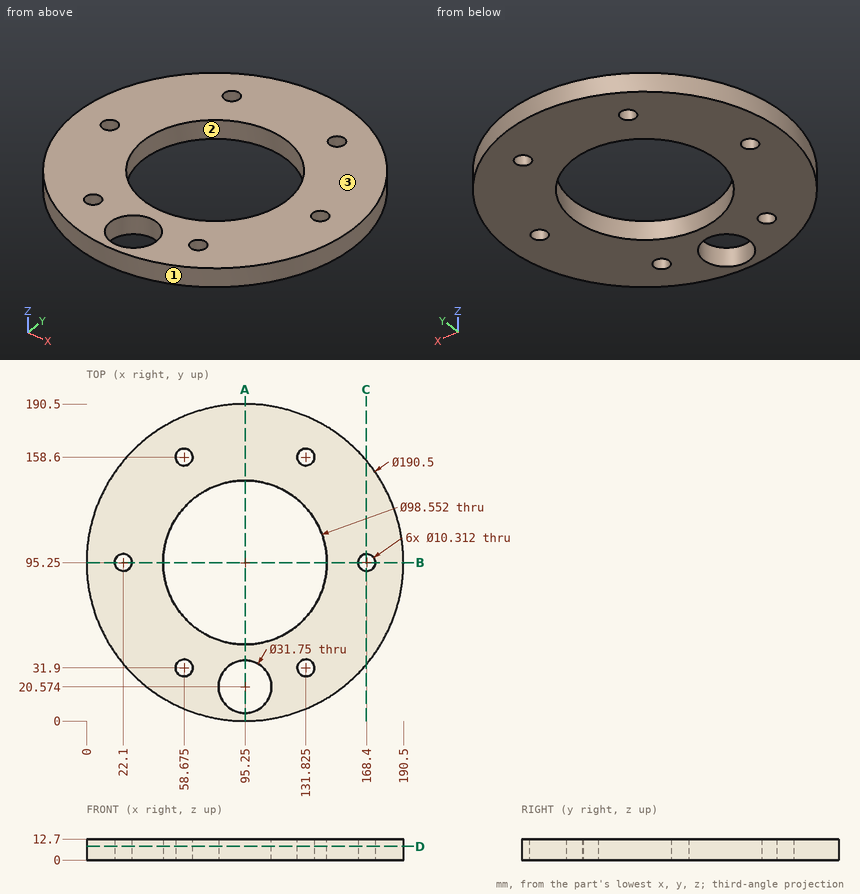
Could you check a few things on this drawing? It's one solid part, dimensions in mm from its lowest x, y, z. Give positions to 0.01 mm unless a question says otherwise; leave off trailing zeros. Loops run counter-clockwise (first coordinate to the right, second up) from the corner with the lowest first, then second, coordinate; pieces in that order, holes last. Notation, with made-up numbers: M -36.75,-37.75 L -28.75,-37.75 A19 cw -28.75,-33.75 Z; hole C 48.25,-33.5 d5. An arc over 180 degrees is marked long. Return JSON: item names as keys, results as strings.
Item 1: Thinking about a two-plate mould opening in X: for the marked faces 1, 2 and 3, which applies, released by +X, released by -X, zero draft, split by the parting line, or undercut?
A:
{"face 1": "split by the parting line", "face 2": "undercut", "face 3": "zero draft"}
Item 2: Imagine slicing it at A-A on x = 95.25. List the corners of the cut face in (y, z) for me.
A:
{"outline": "M 0,0 L 4.7,0 L 4.7,12.7 L 0,12.7 Z; M 36.45,0 L 45.97,0 L 45.97,12.7 L 36.45,12.7 Z; M 144.53,0 L 190.5,0 L 190.5,12.7 L 144.53,12.7 Z"}
Item 3: Imagine slicing it at C-C on x = 168. List the corners of the cut face in (y, z) for me.
A:
{"outline": "M 33.77,0 L 90.11,0 L 90.11,12.7 L 33.77,12.7 Z; M 100.39,0 L 156.73,0 L 156.73,12.7 L 100.39,12.7 Z"}
Item 4: I'm going to push flat-ended pins straight in: pin 1 Ø6 at (x, z) = (124, 2) entering from -Y; pin 2 Ø5 at (y, z) = (112, 11) entering from -X; pin 3 Ø3 at (x, z) = (57, 9) entering from -Y (1 decimal). Where does each tip first touch, or does it pass through?
A:
{"pin 1": "stops at y = 3.55", "pin 2": "stops at x = 1.07", "pin 3": "stops at y = 7.4"}
Item 5: Imagine slicing it at D-D on z = 8.25. State how many separate pieces and enclosed holes the cut face has, then the cut area to 3 significant figures.
A:
{"separate pieces": "1", "enclosed holes": "8", "area": "19,600 mm^2"}
Item 6: Imagine slicing it at B-B on y = 95.25. List the corners of the cut face in (x, z) for me, then the cut area to 3 significant figures.
A:
{"outline": "M 0,0 L 16.94,0 L 16.94,12.7 L 0,12.7 Z; M 27.26,0 L 45.97,0 L 45.97,12.7 L 27.26,12.7 Z; M 144.53,0 L 163.24,0 L 163.24,12.7 L 144.53,12.7 Z; M 173.56,0 L 190.5,0 L 190.5,12.7 L 173.56,12.7 Z", "area": "906 mm^2"}
Item 7: Please list where these lines run through material, in increasing order: line 1 (X direction, y = 30, z = 4.75) (1 decimal); line 2 (X direction, y = 100, z = 3) (1 decimal); line 3 (Y direction, x = 24.5, z = 1.5) (1 decimal).
A:
{"line 1": "x = 25.9 to 53.9, 63.5 to 82.5, 108 to 127, 136.6 to 164.6", "line 2": "x = 0.1 to 20.1, 24.1 to 46.2, 144.3 to 166.4, 170.4 to 190.4", "line 3": "y = 31.5 to 90.7, 99.8 to 159"}
